Check sheet for the drawn part. Datum: minimum x, y, z corner. Units: mm. Coordinates: 2 decimals unless noted, no trailing zeros. Order: outer loops, then holes, each group sorted by start corner. A loop starts at its lowest first (then second) coordinate and runs counter-clockwise, first axis right, second up. Notation, with made-up numbers: (49, 86) - (103, 86) arc R12 cw to (103, 96) - close; hole circle Ø9 at (78, -16). An arc over 180 degrees is marked (long way). Put each result on its own line as item: value.
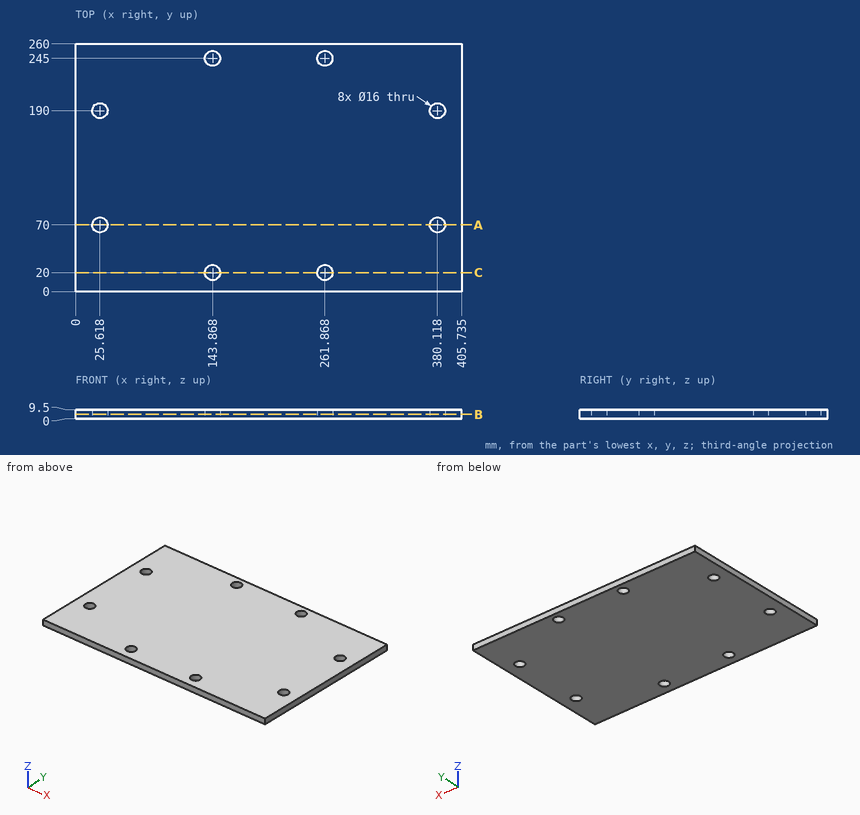
Q1. Depth check by flat-ended pin: pin 1 Ø14.5 at (x, y) = (143.87, 245) entering from +Z. Enter the tip coordinate at first touch or a pass-through.
Answer block:
pin 1: passes through
Q2. Thickness scan on L1, parallel to X at y = 245, z = 6.75 (1 decimal); L2, parallel to X at y = 244, z = 2.5 (1 decimal). Record the ranges inside material, lowest first. Write a range as [from, to].
Answer block:
L1: x = [0, 135.9], [151.9, 253.9], [269.9, 405.7]
L2: x = [0, 135.9], [151.8, 253.9], [269.8, 405.7]
Q3. Section check B-B on z = 4.5. State how many separate pieces and enclosed holes the cut face has, then the cut area to 3 significant figures.
Answer block:
separate pieces: 1
enclosed holes: 8
area: 104,000 mm^2
Q4. Section check C-C on y = 20. Record the boundary of the cut face in (x, z) (1 decimal), then the cut area to 3 significant figures.
Answer block:
outline: (0, 0) - (135.9, 0) - (135.9, 9.5) - (0, 9.5) - close; (151.9, 0) - (253.9, 0) - (253.9, 9.5) - (151.9, 9.5) - close; (269.9, 0) - (405.7, 0) - (405.7, 9.5) - (269.9, 9.5) - close
area: 3,550 mm^2
Q5. Section check A-A on y = 70. Record the boundary of the cut face in (x, z) (1 decimal).
Answer block:
outline: (0, 0) - (17.6, 0) - (17.6, 9.5) - (0, 9.5) - close; (33.6, 0) - (372.1, 0) - (372.1, 9.5) - (33.6, 9.5) - close; (388.1, 0) - (405.7, 0) - (405.7, 9.5) - (388.1, 9.5) - close
